Here's how the part is built. I have some questions about the finished solid (model axes, mm). A direction names the side the tool comes from. Round coordinates to 2 decimals unless told otherwise and drop trailing zeros. Write each loop counter-clockwise with the first axis right and the second up, starting at its lowest first coordinate (ties: lowest second). Pieces come first, ordered by that corner, then holes. Notation, with made-up numbers: (77.5, -37.75) -> (136.5, -37.75) arc R30 ccw to (136.5, -10.75) -> close; hole circle Ø11 at (76, 10). An arc over 180 degrees is marked (long way). Answer in a Markdown table with one row per item.
Autodesk Inventor part; units mm, degrees
ref_plane "YZ Plane" through (0, 0, 0) normal (1, 0, 0) x (0, 1, 0)
ref_plane "XZ Plane" through (0, 0, 0) normal (0, 1, 0) x (-1, 0, 0)
ref_plane "XY Plane" through (0, 0, 0) normal (0, 0, 1) x (1, 0, 0)
sketch "Boceto1" plane through (0, 0, 0) normal (0, 1, 0) x (-1, 0, 0)
  line L0 (8.5, 8.5) -> (-8.5, 8.5)
  line L1 (-8.5, 8.5) -> (-8.5, -8.5)
  line L2 (-8.5, -8.5) -> (8.5, -8.5)
  line L3 (8.5, -8.5) -> (8.5, 8.5)
  line L4 (9.5, 9.5) -> (-9.5, 9.5)
  line L5 (-9.5, 9.5) -> (-9.5, -9.5)
  line L6 (-9.5, -9.5) -> (9.5, -9.5)
  line L7 (9.5, -9.5) -> (9.5, 9.5)
  point P0 (0, 0)
  point P1 (8.5, 0)
  point P2 (0, -8.5)
  dimension "d0" = 17
  dimension "d1" = 17
  dimension "d2" = 1
  dimension "d3" = 1
  dimension "d4" = 1
  dimension "d5" = 1
extrude "Extrusión1" add sketch "Boceto1" along normal blind 15
extrude "Extrusión2" add sketch "Boceto1" along normal blind 1 contours L3 L2 L1 L0
properties part number "cubo"
1) I want a section at B-B, the plane x = 0. List the corners of the cut face in (y, z) for me, and give its area (3 significant figures).
Response:
| item | result |
|---|---|
| outline | (0, -9.5) -> (15, -9.5) -> (15, -8.5) -> (1, -8.5) -> (1, 8.5) -> (15, 8.5) -> (15, 9.5) -> (0, 9.5) -> close |
| area | 47.0 mm^2 |
2) I want a section at A-A, the plane y = 2.75. List the corners of the cut face in (x, z) for me.
Response:
| item | result |
|---|---|
| outline | (-9.5, -9.5) -> (9.5, -9.5) -> (9.5, 9.5) -> (-9.5, 9.5) -> close; hole (-8.5, -8.5) -> (8.5, -8.5) -> (8.5, 8.5) -> (-8.5, 8.5) -> close |
3) Which directions (+Z, -Z, +X, -X, +Y, -Y) give clear straight access to the entire face, cutting with the end or side of a thin tool? Please do faces 1 (the face through (0, 1, 0)), 2 (the face through (1, 15, -9)).
Response:
| item | result |
|---|---|
| face 1 | +Y |
| face 2 | +Z, -Z, +X, -X, +Y |
4) I need wall thicknesses on line 1 (Z direction, x = -5, y = 11.75); line 2 (Y direction, x = -3.5, z = 0.5). Which ranges of each line are inside material? Lowest first, please. Write a range as [from, to].
Response:
| item | result |
|---|---|
| line 1 | z = [-9.5, -8.5], [8.5, 9.5] |
| line 2 | y = [0, 1] |
5) For pin 1 (5 mm diameter, centred on x = -2.5, z = 2, fed in from +Y), with a flat end and sliding along its axis, tell me the tip position at first contact or that it passes through.
Response:
| item | result |
|---|---|
| pin 1 | stops at y = 1 |
6) I want a section at C-C, the plane z = 2. List the corners of the cut face in (x, y) for me, and give its area (3 significant figures).
Response:
| item | result |
|---|---|
| outline | (-9.5, 0) -> (9.5, 0) -> (9.5, 15) -> (8.5, 15) -> (8.5, 1) -> (-8.5, 1) -> (-8.5, 15) -> (-9.5, 15) -> close |
| area | 47.0 mm^2 |
7) We'd pull the mould along X, two halves only. Please class faces 3 (the face through (-9.5, 7, 0)), 4 (the face through (0, 7, -9.5)), 5 (the face through (0, 8, 8.5)), 6 (the face through (-8.5, 8, 0)): +X half, -X half, draft (parallel to the pull), parting line (faces both ways), or undercut.
Response:
| item | result |
|---|---|
| face 3 | -X half |
| face 4 | draft |
| face 5 | undercut |
| face 6 | undercut |
